Geometry: final body of the model. Coordinates: model frame, mm. Coordinates: 2 decimals unless noted, no trailing zeros. Write each loop counter-clockwise with the first axis right and the second up, starting at its lowest first coordinate (ties: lowest second). Pieces come first, ordered by that corner, then holes.
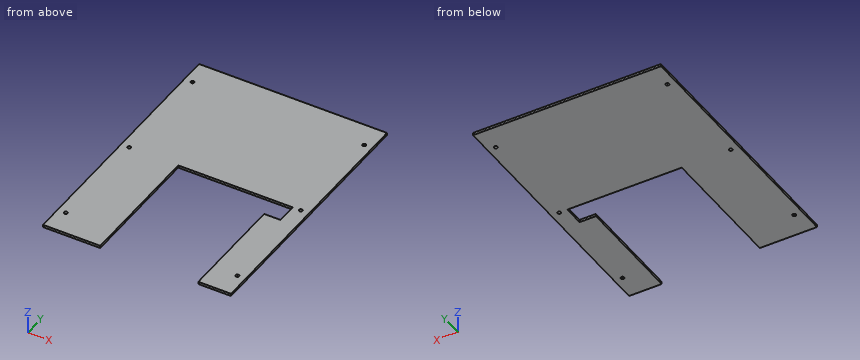
from build123d import *

# Parameters (mm, degrees)
F1_W     = 230
F1_H     = 320
F2_DEPTH = 3
F4_D     = 4.2
F4_DEPTH = 4
F4_TIP   = 1.2618073
F5_W     = 120
F5_H     = 160
F6_DEPTH = 25
F7_W     = 20
F7_H     = 25
F8_DEPTH = 3


# Not quite as in the source:
# - a pattern or mirror of a feature is missing from the dataset's text; its kind, count and spacing are read off the source's solid


with BuildPart() as f2:
    # F1 (on Top) → F2 (new body)
    with BuildSketch(Plane.XY):
        Rectangle(F1_W, F1_H)
    extrude(amount=F2_DEPTH)

    # F4
    with Locations(Plane.XY.offset(3)):
        with Locations((-105, 130), (-105, 0), (-105, -130)):
            f4 = Hole(F4_D / 2, depth=F4_DEPTH)
            with Locations((0, 0, -(F4_DEPTH + F4_TIP / 2))):  # 118° drill point
                Cone(0, F4_D / 2, F4_TIP, mode=Mode.SUBTRACT)

    # F4_copies: F4 across plane
    add(f4.mirror(Plane(origin=(0, 0, 0), x_dir=(0, 0, 1), z_dir=(1, 0, 0))), mode=Mode.SUBTRACT)

    # F5 (on face) → F6 (cut)
    with BuildSketch(Plane.XY.offset(3)):
        with Locations((15, -80)):
            Rectangle(F5_W, F5_H)
    extrude(amount=-F6_DEPTH, mode=Mode.SUBTRACT)

    # F7 (on face) → F8 (cut, through all)
    with BuildSketch(Plane.XY.offset(3)):
        with Locations((85, -12.5)):
            Rectangle(F7_W, F7_H)
    extrude(amount=-F8_DEPTH, mode=Mode.SUBTRACT)


solid = f2.part
Item 1: Section C-C, the plane x = 35. Output: boundary loops of the cut face in (y, z).
Derived:
outline: (0, 0) - (160, 0) - (160, 3) - (0, 3) - close
Item 2: Section B-B, the plane z = 1.7. Output: boundary loops of the cut face in (x, y).
Derived:
outline: (-115, -160) - (-45, -160) - (-45, 0) - (95, 0) - (95, -25) - (75, -25) - (75, -160) - (115, -160) - (115, 160) - (-115, 160) - close; hole circle Ø4.2 at (-105, -130); hole circle Ø4.2 at (-105, 0); hole circle Ø4.2 at (-105, 130); hole circle Ø4.2 at (105, -130); hole circle Ø4.2 at (105, 0); hole circle Ø4.2 at (105, 130)
Item 3: Material intervals for probe 1 along Y at (x, z) = (-105, 1.1); probe 2 along Y at (x, z) = (91, 1.25); probe 3 along X at (y, z) = (-83.5, 2.1), sorted ascending.
Derived:
probe 1: y = -160 to -132.1, -127.9 to -2.1, 2.1 to 127.9, 132.1 to 160
probe 2: y = -160 to -25, 0 to 160
probe 3: x = -115 to -45, 75 to 115
Item 4: Section A-A, the plane y = -49. Output: boundary loops of the cut face in (x, z), plus the area to 3 significant figures.
Derived:
outline: (-115, 0) - (-45, 0) - (-45, 3) - (-115, 3) - close; (75, 0) - (115, 0) - (115, 3) - (75, 3) - close
area: 330 mm2
